Geometry check sheet. Reference: drawing and pictorial views, mm from the part's lowest x, y, z. A direction names the side the tool comes from. Round coordinates to 2 decimals unless told otherwise and drop trailing zeros. Write each loop counter-clockwise with the first axis right and the second up, starting at its lowest first coordinate (ties: lowest second). Pieces come first, ordered by that corner, then holes. Notation, with made-up numbers: (71, 89) -> (93, 89) arc R13 cw to (93, 101) -> close; hole circle Ø5 at (-5.5, 60.25). An arc over 180 degrees is marked (long way). Answer as a JSON object with one key per item and string values. Group by question number.
(1) Sectioned sample at C-C on y = 502.5. Record the cut outline in (x, z), and give its area (3 significant figures).
(2) Sectioned sample at B-B on z = 19. Record the cut outline in (x, y), and give its area (3 significant figures).
(3) Scan lines: L1, parallel to Y at x = 69.5, z = 13.5; L2, parallel to Y at x = 12.5, z = 12. Record each from-to range of solid material in increasing order. Write a range as from..to.
(4) Sectioned sample at A-A on x = 40. Record the cut outline in (y, z).
(5) Set-up check for the marked faces 1, 2, 3, 4 and 5: record each of +Z, -Z, +X, -X, +Y, -Y from which the full face is reachable in a straight line by a thin tool's end or side.
(6) Gauge pin test, flat ends, axial feed: pin 1 Ø12 at (x, z) = (55.5, 33) entering from +Y; pin 2 Ø8 at (x, z) = (27, 22.5) entering from -Y; pin 3 Ø6.5 at (x, z) = (45.5, 29) entering from -Y; pin 4 Ø4 at (y, z) = (517.5, 19.5) entering from +X. Record the tip position at first contact, or that the pin passes through.
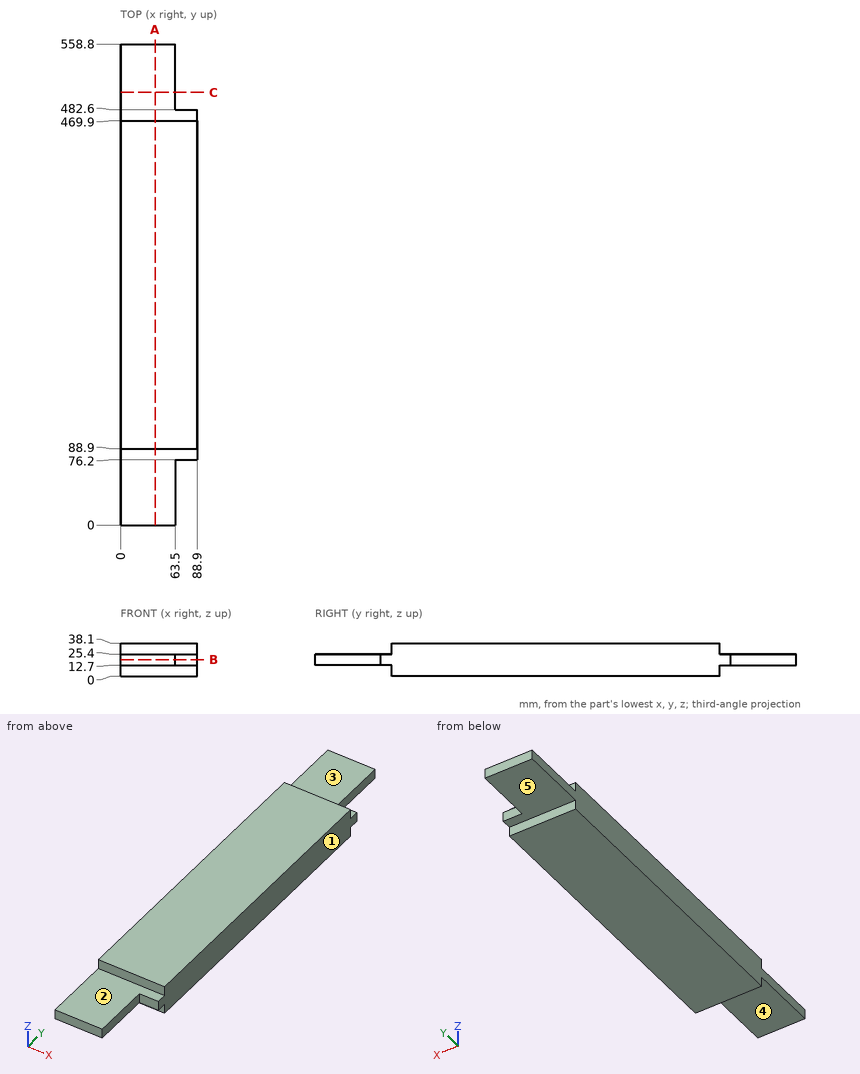
Computed values:
{
 "1": {"outline": "(0, 12.7) -> (63.5, 12.7) -> (63.5, 25.4) -> (0, 25.4) -> close", "area": "806 mm2"},
 "2": {"outline": "(0, 0) -> (63.5, 0) -> (63.5, 76.2) -> (88.9, 76.2) -> (88.9, 482.6) -> (63.5, 482.6) -> (63.5, 558.8) -> (0, 558.8) -> close", "area": "45,800 mm2"},
 "3": {"L1": "76.2..482.6", "L2": "88.9..469.9"},
 "4": {"outline": "(0, 12.7) -> (88.9, 12.7) -> (88.9, 0) -> (469.9, 0) -> (469.9, 12.7) -> (558.8, 12.7) -> (558.8, 25.4) -> (469.9, 25.4) -> (469.9, 38.1) -> (88.9, 38.1) -> (88.9, 25.4) -> (0, 25.4) -> close"},
 "5": {"face 1": "+Z, -Z, +X, +Y, -Y", "face 2": "+Z, +X, -X, -Y", "face 3": "+Z, +X, -X, +Y", "face 4": "-Z, +X, -X, -Y", "face 5": "-Z, +X, -X, +Y"},
 "6": {"pin 1": "y = 469.9", "pin 2": "y = 0", "pin 3": "y = 88.9", "pin 4": "x = 63.5"}
}
